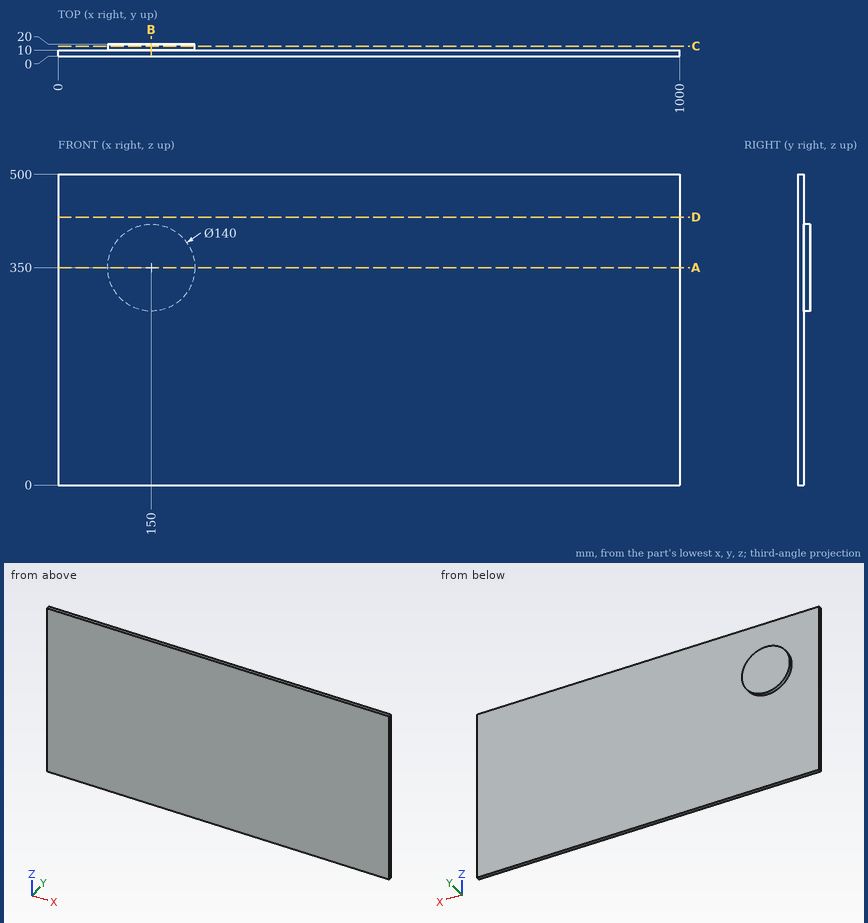
Geometry: see drawing. Coordinates: mm, zero at the bounding-box minimum. Give positions to 0.01 mm unless a question says otherwise; leave off trailing zeros. Loops run counter-clockwise (first coordinate to the right, second up) from the corner with the lowest first, then second, coordinate; pieces in that order, holes last. Notation, with made-up numbers: (78.5, -0.5) -> (95.5, -0.5) arc R8 cw to (95.5, 12.5) -> close; hole circle Ø6 at (-2.5, -10.5). An arc over 180 degrees is marked (long way). Put each result on its own line as item: value.
1. Cut plane A-A (z = 350). Return the cut outline in (x, y), plus the area to 3 significant figures.
Taken from the geometry:
outline: (0, 0) -> (1000, 0) -> (1000, 10) -> (220, 10) -> (220, 20) -> (80, 20) -> (80, 10) -> (0, 10) -> close
area: 11,400 mm2
2. Ray query, line 1 along Y through (x, z) = (64, 253.5); line 2 along X through (y, z) = (15, 403.5); line 3 along Z through (x, y) = (187, 16). Return the intervals inside material, ascending. Write a range as [from, to].
Taken from the geometry:
line 1: y = [0, 10]
line 2: x = [104.86, 195.14]
line 3: z = [290.58, 409.42]
3. Cut plane B-B (x = 150). Return the cut outline in (y, z).
Taken from the geometry:
outline: (0, 0) -> (10, 0) -> (10, 280) -> (20, 280) -> (20, 420) -> (10, 420) -> (10, 500) -> (0, 500) -> close
4. Cut plane C-C (y = 16.5). Return the cut outline in (x, z), plus the area to 3 significant figures.
Taken from the geometry:
outline: circle Ø140 at (150, 350)
area: 15,400 mm2
5. Pin query (flat end, axial travel): P1, Ø1.5, axis at y = 11, z = 141, coming from the +X side; P2, Ø3, axis at x = 440.5, z = 408.5, coming from the +Y side. Return the tip coordinate at first contact, or that it passes through.
Taken from the geometry:
P1: passes through
P2: stops at y = 10
6. Cut plane D-D (z = 431.5). Return the cut outline in (x, y), plus the area to 3 significant figures.
Taken from the geometry:
outline: (0, 0) -> (1000, 0) -> (1000, 10) -> (0, 10) -> close
area: 10,000 mm2
